Part model, mm, in its own coordinate system. A direction names the side the tool comes from. Give positions to 0.01 mm unless a question says otherwise; leave off trailing zeros. Write each loop counter-clockwise with the first axis right and the second up, starting at its lowest first coordinate (ties: lowest second). Pieces come first, ordered by that corner, then holes. Notation, with made-up numbers: M -1.5,50.5 L 45.5,50.5 A17 ccw 45.5,75.5 Z; hole C 17,10 d11. An arc over 180 degrees is marked long. Answer as CSV lines item,"result". Start each with the question number.
1) Slice it at B-B, the plane y = 0. Give the cut face in (x, z), plus the area to 3 significant figures.
2) Tool access for faces 5 (the conical face through (-50.69, -11.5, 2.42)), 6 (the flat face through (89, 12.5, 17)), 7 (the cylindrical face through (33.944, -36.713, 5.972)): list every direction of +Z, -Z, +X, -X, +Y, -Y with a clear straight run to the whole face (end or side of a thin tool).
3) Slice it at C-C, the plane z = 17. Give the cut face in (x, y).
4) Slice it at A-A, the plane x = -75.5. Give the cut face in (y, z).
5) Pin check, flat tips, straight feed: pin 1 Ø11 at (x, z) = (90.5, 17) entering from +Y; pin 2 Ø11 at (x, z) = (91, 18) entering from -Y. Stop position of each tip, or through.
6) Wall check: line 1 along X through (y, z) = (0, 15); line 2 along X through (y, z) = (0, 5.25); line 3 along Z through (x, y) = (-75.5, -61.6). Give the ranges that are in metal, low to high. Write a range as from..to.
7) Mould opens along Y. For faces 1 (the cylindrical face through (-91.22, 59.49, 9.86)), 2 (the flat face through (-45, -59, 12)), 3 (the flat face through (95.5, -1, 10)), 4 (the conical face through (15.38, 49.65, 2.42)) say: pulls with the +Y half, pulls with the -Y half, needs draft (parallel to the pull), parting line crosses it, or undercut.
8) Slice it at D-D, the plane x = 70.5. Give the cut face in (y, z).
```python
from build123d import *

# Parameters (mm, degrees)
BOSS_EXTRUDE1_DEPTH      = 20
SKETCH2_R                = 55
CUT_EXTRUDE1_DEPTH       = 117.688688398
SHELL1_T                 = -5
FILLET1_R                = 2
CIRPATTERN1_COUNT        = 3
FILLET1_OF_CIRPATTERN1_R = 2
SKETCH5_R                = 10
CUT_EXTRUDE2_DEPTH       = 117.688688398
CUT_EXTRUDE3_DEPTH       = 117.688688398
CUT_EXTRUDE3_DEPTH_BACK  = 117.688688398
SKETCH6_R                = 3.5
SKETCH7_W                = 10
SKETCH7_H                = 25
BOSS_EXTRUDE2_DEPTH      = 20


with BuildPart() as part:
    # Sketch1 → Boss-Extrude1 (new body)
    with BuildSketch(Plane.XY):
        with BuildLine():
            Line((-80.5, 64), (80.5, 64))
            ThreePointArc((80.5, 64), (91.106601718, 59.606601718), (95.5, 49))
            Line((95.5, 49), (95.5, -49))
            ThreePointArc((95.5, -49), (91.106601718, -59.606601718), (80.5, -64))
            Line((80.5, -64), (-80.5, -64))
            ThreePointArc((-80.5, -64), (-91.106601718, -59.606601718), (-95.5, -49))
            Line((-95.5, -49), (-95.5, 49))
            ThreePointArc((-95.5, 49), (-91.106601718, 59.606601718), (-80.5, 64))
        make_face()
    extrude(amount=BOSS_EXTRUDE1_DEPTH)

    # Sketch2 → Cut-Extrude1 (cut, through all)
    with BuildSketch(Plane.XY.offset(20)):
        Circle(SKETCH2_R)
    extrude(amount=-CUT_EXTRUDE1_DEPTH, mode=Mode.SUBTRACT)

    # Shell1
    shell1_openings = [part.faces().sort_by_distance(p)[0] for p in [
        (0, 61.700760995, 20),
    ]]
    offset(amount=SHELL1_T, openings=shell1_openings)

    # Sweep1: sweep along a path in Sketch4
    with BuildLine(Plane.XY) as sweep1_path:
        ThreePointArc((0, 50), (15, 47.696960071), (28.618176043, 41))
    # Sketch3 → Sweep1 (sweep)
    with BuildSketch(Plane(origin=(0, 0, 0), x_dir=(0, 0, -1), z_dir=(1, 0, 0))):
        Polygon((0, 55), (-12, 55), (-8, 50), (-4, 50), align=None)
    sweep1 = sweep(path=sweep1_path.line)

    # Fillet1
    fillet1_edges = [part.edges().sort_by_distance(p)[0] for p in [
        (28.618176043, 41, 6),
        (0, 50, 6),
    ]]
    fillet(fillet1_edges, radius=FILLET1_R)

    # CirPattern1: Sweep1 ×3 about axis
    cirpattern1_axis = Axis((0, 0, 0), (0, 0, 1))
    for i in range(1, CIRPATTERN1_COUNT):
        add(sweep1.rotate(cirpattern1_axis, i * 360 / CIRPATTERN1_COUNT))

    # Fillet1 of CirPattern1
    fillet1_of_cirpattern1_edges = [part.edges().sort_by_distance(p)[0] for p in [
        (-49.816129576, 4.284067463, 6),
        (-43.301270189, -25, 6),
        (21.197953534, -45.284067463, 6),
        (43.301270189, -25, 6),
    ]]
    fillet(fillet1_of_cirpattern1_edges, radius=FILLET1_OF_CIRPATTERN1_R)

    # Sketch5 → Cut-Extrude2 (cut, through all)
    with BuildSketch(Plane(origin=(0, 0, 0), x_dir=(-1, 0, 0), z_dir=(0, 0, -1))):
        with Locations((-70.5, -39)):
            Circle(SKETCH5_R)
    extrude(amount=-CUT_EXTRUDE2_DEPTH, mode=Mode.SUBTRACT)

    # Sketch6 → Cut-Extrude3 (cut, two sides: drawn at the far end of the back side and taken through both)
    with BuildSketch(Plane(origin=(0, 0, 0), x_dir=(1, 0, 0), z_dir=(0, 1, 0)).offset(-CUT_EXTRUDE3_DEPTH_BACK)):
        with Locations(Location((-75.5, -11, 0), (0, 0, 270))):
            Circle(SKETCH6_R)
    extrude(amount=CUT_EXTRUDE3_DEPTH + CUT_EXTRUDE3_DEPTH_BACK, mode=Mode.SUBTRACT)

    # Sketch7 → Boss-Extrude2 (add)
    with BuildSketch(Plane.XY.offset(5)):
        with Locations((90.5, 0)):
            Rectangle(SKETCH7_W, SKETCH7_H)
    extrude(amount=BOSS_EXTRUDE2_DEPTH)


solid = part.part
```
Found:
1,outline,"M -95.5,0 L -55,0 L -50,4 L -50,8 L -55,12 L -55,20 L -60,20 L -60,5 L -90.5,5 L -90.5,20 L -95.5,20 Z; M 55,0 L 95.5,0 L 95.5,25 L 85.5,25 L 85.5,5 L 60,5 L 60,20 L 55,20 Z"
1,area,"870 mm²"
2,face 5,"-Z"
2,face 6,"+Z"
2,face 7,"+Z, -Z"
3,outline,"M -95.5,-49 A15 ccw -80.5,-64 L 80.5,-64 A15 ccw 95.5,-49 L 95.5,49 A15 ccw 80.5,64 L -80.5,64 A15 ccw -95.5,49 Z; hole M -90.5,-49 A10 ccw -80.5,-59 L -10.91,-59 A60 cw -10.91,59 L -80.5,59 A10 ccw -90.5,49 Z; hole C 0,0 d110; hole M 10.91,-59 L 80.5,-59 A10 ccw 90.5,-49 L 90.5,-12.5 L 85.5,-12.5 L 85.5,12.5 L 90.5,12.5 L 90.5,49 A10 ccw 80.5,59 L 10.91,59 A60 cw Z"
4,outline,"M -64,0 L 64,0 L 64,7.5 L 59,7.5 L 59,5 L -59,5 L -59,7.5 L -64,7.5 Z; M -64,14.5 L -59,14.5 L -59,20 L -64,20 Z; M 59,14.5 L 64,14.5 L 64,20 L 59,20 Z"
5,pin 1,"y = 63.31"
5,pin 2,"y = -63.14"
6,line 1,"-95.5..-90.5, -60..-55, 55..60, 85.5..95.5"
6,line 2,"-95.5..-90.5, -60..-50, 55..60, 85.5..95.5"
6,line 3,"0..7.5, 14.5..20"
7,face 1,"pulls with the +Y half"
7,face 2,"undercut"
7,face 3,"needs draft"
7,face 4,"undercut"
8,outline,"M -64,0 L -49,0 L -49,5 L -59,5 L -59,20 L -64,20 Z; M -29,0 L 64,0 L 64,20 L 59,20 L 59,5 L -29,5 Z"
